from build123d import *

# Parameters (mm, degrees)
ESQUISSE1_R             = 10.75
ESQUISSE1_R_2           = 2.75
BASE_EXTRUSION_DEPTH    = 8
ESQUISSE2_R             = 12.75
ESQUISSE2_R_2           = 2.75
BOSS_EXTRU_1_DEPTH      = 62
ENL_V_MAT_EXTRU_1_REACH = 74.285


with BuildPart() as part:
    # Esquisse1 → Base-Extrusion (new body)
    with BuildSketch(Plane.XY):
        Circle(ESQUISSE1_R)
        Circle(ESQUISSE1_R_2, mode=Mode.SUBTRACT)
    extrude(amount=BASE_EXTRUSION_DEPTH)

    # Esquisse2 → Boss.-Extru.1 (add)
    with BuildSketch(Plane.XY.offset(8)):
        Circle(ESQUISSE2_R)
        Circle(ESQUISSE2_R_2, mode=Mode.SUBTRACT)
    extrude(amount=BOSS_EXTRU_1_DEPTH)

    # Esquisse4 → Enlèv. mat.-Extru.1 (cut, up to next)
    with BuildSketch(Plane.XY.offset(70), mode=Mode.PRIVATE) as enl_v_mat_extru_1_sk1:
        with BuildLine():
            Line((7.158163625, 10.671606885), (6.672416375, 9.977041632))
            Line((6.672416375, 9.977041632), (7.082156576, 9.690488028))
            Line((7.082156576, 9.690488028), (7.567903827, 10.385053282))
            ThreePointArc((7.567903827, 10.385053282), (7.364427601, 10.530323172), (7.158163625, 10.671606885))
        make_face()
    enl_v_mat_extru_1_tool1 = extrude(enl_v_mat_extru_1_sk1.sketch, amount=-ENL_V_MAT_EXTRU_1_REACH, mode=Mode.PRIVATE) & part.part
    # Esquisse4 → Enlèv. mat.-Extru.1 (cut, up to next)
    with BuildSketch(Plane.XY.offset(70), mode=Mode.PRIVATE) as enl_v_mat_extru_1_sk2:
        with BuildLine():
            Line((5.662800849, -11.534954987), (5.30416332, -10.767002901))
            Line((5.30416332, -10.767002901), (4.851130519, -10.978571523))
            Line((4.851130519, -10.978571523), (5.209768049, -11.746523608))
            ThreePointArc((5.209768049, -11.746523608), (5.437313576, -11.642942973), (5.662800849, -11.534954987))
        make_face()
    enl_v_mat_extru_1_tool2 = extrude(enl_v_mat_extru_1_sk2.sketch, amount=-ENL_V_MAT_EXTRU_1_REACH, mode=Mode.PRIVATE) & part.part
    # Esquisse4 → Enlèv. mat.-Extru.1 (cut, up to next)
    with BuildSketch(Plane.XY.offset(70), mode=Mode.PRIVATE) as enl_v_mat_extru_1_sk3:
        with BuildLine():
            Line((-12.820964474, 0.863348101), (-11.976579695, 0.78996127))
            Line((-11.976579695, 0.78996127), (-11.933287096, 1.288083495))
            Line((-11.933287096, 1.288083495), (-12.777671875, 1.361470326))
            ThreePointArc((-12.777671875, 1.361470326), (-12.801741178, 1.112619801), (-12.820964474, 0.863348101))
        make_face()
    enl_v_mat_extru_1_tool3 = extrude(enl_v_mat_extru_1_sk3.sketch, amount=-ENL_V_MAT_EXTRU_1_REACH, mode=Mode.PRIVATE) & part.part
    add(enl_v_mat_extru_1_tool1.solids().sort_by_distance((7.120625, 10.181712, 70))[0], mode=Mode.SUBTRACT)
    add(enl_v_mat_extru_1_tool2.solids().sort_by_distance((5.257309, -11.257498, 70))[0], mode=Mode.SUBTRACT)
    add(enl_v_mat_extru_1_tool3.solids().sort_by_distance((-12.377934, 1.075786, 70))[0], mode=Mode.SUBTRACT)


solid = part.part
Geometry check sheet. Reference: the model listing, model coordinates, mm. A direction names the side the tool comes from. Round coordinates to 2 decimals unless told otherwise and drop trailing zeros. Loops run counter-clockwise (first coordinate to the right, second up) from the corner with the lowest first, then second, coordinate; pieces in that order, holes last. Notation, with made-up numbers: (69, 58) - (116, 58) arc R37 cw to (116, 97) - close; hole circle Ø1 at (36.25, 64). An arc over 180 degrees is marked (long way). One line per question, with ' | ' between items. Start each with the question number.
1. Depth check by flat-ended pin: pin 1 (1 mm diameter, centred on y = -2.5, z = 63, fed in from +X); pin 2 (1.5 mm diameter, centred on x = 4, z = 10.5, fed in from -Y); pin 3 (1 mm diameter, centred on x = -1, z = 22, fed in from +Y); pin 4 (5 mm diameter, centred on x = 0, y = 0, fed in from +Z) (1 decimal). Enter the tip coordinate at first touch or a pass-through.
2. Scan lines: line 1 (Y direction, x = 0, z = 39); line 2 (Y direction, x = -2.5, z = 31); line 3 (X direction, y = -1, z = 34). Record each from-to range of solid material in increasing order. Write a range as [from, to].
3. Cross-section at C-C on z = 60.5. Record the cut outline in (x, y).
4. Cross-section at D-D on y = -5.5. Record the cut outline in (x, z), then the cut area to 3 significant figures.
5. Cross-section at A-A on x = 0. Record the cut outline in (y, z), then the cut area to 3 significant figures.
6. Tool access check on faces 1 (the face through (-1.4, 10.66, 3.94)), 2 (the face through (2.2, -2.2, 0)). Record the directions out of +Z, -Z, +X, -X, +Y, -Y that give a thin tool (end or side, any length) a straight path to the whole face; none if there is none.
Taken from the geometry:
1) pin 1: x = 12.59 | pin 2: y = -12.33 | pin 3: y = 12.74 | pin 4: through
2) line 1: [-12.75, -2.75], [2.75, 12.75] | line 2: [-12.5, -1.15], [1.15, 12.5] | line 3: [-12.71, -2.56], [2.56, 12.71]
3) outline: (-12.72, 0.85) arc R12.75 ccw to (5.17, -11.66) - (4.85, -10.98) - (5.3, -10.77) - (5.62, -11.44) arc R12.75 ccw to (7.51, 10.3) - (7.08, 9.69) - (6.67, 9.98) - (7.1, 10.59) arc R12.75 ccw to (-12.68, 1.35) - (-11.93, 1.29) - (-11.98, 0.79) - close; hole circle Ø5.5 at (0, 0)
4) outline: (-11.5, 8) - (-9.24, 8) - (-9.24, 0) - (9.24, 0) - (9.24, 8) - (11.5, 8) - (11.5, 70) - (-11.5, 70) - close | area: 1,570 mm²
5) outline: (-12.75, 8) - (-10.75, 8) - (-10.75, 0) - (-2.75, 0) - (-2.75, 70) - (-12.75, 70) - close; (2.75, 0) - (10.75, 0) - (10.75, 8) - (12.75, 8) - (12.75, 70) - (2.75, 70) - close | area: 1,370 mm²
6) face 1: -Z | face 2: -Z, +X, -X, +Y, -Y
